Source: CAD feature listing. Evaluate the final solid. Frame: model axes, mm. Give positions to 0.01 mm unless a question says otherwise; leave off trailing zeros. Loops run counter-clockwise (first coordinate to the right, second up) from the corner with the lowest first, then second, coordinate; pieces in that order, holes last.
```python
from build123d import *

# Parameters (mm, degrees)
SALIENTE_EXTRUIR1_DEPTH = 25.4
CROQUIS2_R              = 3
CORTAR_EXTRUIR2_DEPTH   = 26.4


with BuildPart() as part:
    # Croquis1 → Saliente-Extruir1 (new body)
    with BuildSketch(Plane(origin=(0, 0, 0), x_dir=(1, 0, 0), z_dir=(0, 1, 0))):
        Polygon((115.470053838, -200), (230.940107676, 0), (115.470053838, 200), (-115.470053838, 200), (-230.940107676, 0), (-115.470053838, -200), align=None)
        Polygon((127.017059222, 0), (63.508529611, 110), (-63.508529611, 110), (-127.017059222, 0), (-63.508529611, -110), (63.508529611, -110), align=None, mode=Mode.SUBTRACT)
    extrude(amount=SALIENTE_EXTRUIR1_DEPTH)

    # Croquis2 → Cortar-Extruir2 (cut, through all)
    with BuildSketch(Plane(origin=(0, 25.4, 0), x_dir=(1, 0, 0), z_dir=(0, 1, 0))):
        with Locations((0, -184.3)):
            Circle(CROQUIS2_R)
        with Locations((-22.5, -184.3)):
            Circle(CROQUIS2_R)
        with Locations((22.5, -184.3)):
            Circle(CROQUIS2_R)
        with Locations((-148.358481917, 111.635571585)):
            Circle(CROQUIS2_R)
        with Locations((-159.608481917, 92.15)):
            Circle(CROQUIS2_R)
        with Locations((-170.858481917, 72.664428415)):
            Circle(CROQUIS2_R)
        with Locations((170.858481917, 72.664428415)):
            Circle(CROQUIS2_R)
        with Locations((159.608481917, 92.15)):
            Circle(CROQUIS2_R)
        with Locations((148.358481917, 111.635571585)):
            Circle(CROQUIS2_R)
    extrude(amount=-CORTAR_EXTRUIR2_DEPTH, mode=Mode.SUBTRACT)


solid = part.part
```
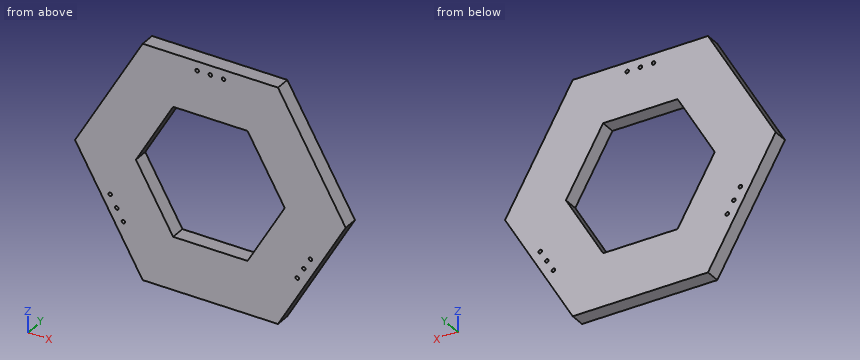
(1) Section A-A, the plane x = -90. Return the cut outline in (y, z).
A:
outline: (0, -200) - (25.4, -200) - (25.4, -64.12) - (0, -64.12) - close; (0, 64.12) - (25.4, 64.12) - (25.4, 200) - (0, 200) - close
(2) First-contact query: pin 1 (3.5 mm diameter, centred on x = 170.86, z = -72.66, fed in from -Y); pin 2 (1 mm diameter, centred on x = 151, y = 4, fed in from -Z); pin 3 (5 mm diameter, centred on y = 5.5, z = -105.5, fed in from -X); pin 4 (6 mm diameter, centred on y = 13, z = 118, fed in from -X). Flat tips, straight axial feed; report the tip coordinate or a pass-through.
A:
pin 1: passes through
pin 2: stops at z = -139.33
pin 3: stops at x = -171.47
pin 4: stops at x = -164.54
(3) Ray query, line 1 along Z through (x, y) = (-22.5, 15); line 2 along X through (y, z) = (10.75, -92.15); line 3 along X through (y, z) = (18, -94). Return the intervals inside material, ascending.
A:
line 1: z = -200 to -110, 110 to 181.3, 187.3 to 200
line 2: x = -177.74 to -162.61, -156.61 to -73.81, 73.81 to 156.61, 162.61 to 177.74
line 3: x = -176.67 to -161.97, -157.25 to -72.75, 72.75 to 157.25, 161.97 to 176.67
(4) Section C-C, the plane z = 151. Return the cut outline in (x, y), then the cut area to 3 significant figures.
A:
outline: (-143.76, 0) - (143.76, 0) - (143.76, 25.4) - (-143.76, 25.4) - close
area: 7,300 mm2
(5) Section B-B, the plane y = 11.25. Count the separate pieces of the cut face and the enclosed holes in it, then the cut area to 3 significant figures.
A:
separate pieces: 1
enclosed holes: 10
area: 96,400 mm2
(6) Section D-D, the plane x = -188. Return the cut outline in (y, z), then the cut area to 3 significant figures.
A:
outline: (0, -74.37) - (25.4, -74.37) - (25.4, 74.37) - (0, 74.37) - close
area: 3,780 mm2
